```python
from build123d import *

# Parameters (mm, degrees)
CROQUIS1_W              = 900
CROQUIS1_H              = 1047
SALIENTE_EXTRUIR1_DEPTH = 2113
VACIADO2_T              = -10
CROQUIS2_W              = 880
CROQUIS2_H              = 2093
SALIENTE_EXTRUIR2_DEPTH = 5
CORTAR_EXTRUIR1_DEPTH   = 2
SALIENTE_EXTRUIR3_DEPTH = 300


with BuildPart() as part:
    # Croquis1 → Saliente-Extruir1 (new body)
    with BuildSketch(Plane(origin=(0, 0, 0), x_dir=(1, 0, 0), z_dir=(0, 1, 0))):
        Rectangle(CROQUIS1_W, CROQUIS1_H)
    extrude(amount=SALIENTE_EXTRUIR1_DEPTH)

    # Vaciado2
    vaciado2_openings = [part.faces().sort_by_distance(p)[0] for p in [
        (0, 1056.5, 523.5),
    ]]
    offset(amount=VACIADO2_T, openings=vaciado2_openings, kind=Kind.INTERSECTION)

    # Croquis2 → Saliente-Extruir2 (add)
    with BuildSketch(Plane.XY.offset(523.5)):
        with Locations((0, 1056.5)):
            Rectangle(CROQUIS2_W, CROQUIS2_H)
    extrude(amount=-SALIENTE_EXTRUIR2_DEPTH)

    # Croquis3 → Cortar-Extruir1 (cut)
    with BuildSketch(Plane.XY.offset(523.5)):
        Polygon((-136.509991439, 890.520139483), (155.469712472, 890.520139483), (9.479860517, 1243.170950701), align=None)
        Polygon((-63.176808732, 920.19459615), (-42.169545822, 1034.041849102), (9.479860517, 1064.169920858), (9.479860517, 1169.411963853), (65.966344659, 1064.169920858), (-12.532301764, 1019.623730372), (-63.176808732, 898.913148296), align=None, mode=Mode.SUBTRACT)
    extrude(amount=-CORTAR_EXTRUIR1_DEPTH, mode=Mode.SUBTRACT)

    # Croquis4 → Saliente-Extruir3 (add)
    with BuildSketch(Plane.XZ):
        with BuildLine():
            Line((-454.35645152, 548.5), (454.35645152, 548.5))
            ThreePointArc((454.35645152, 548.5), (468.953644638, 542.453644638), (475, 527.85645152))
            Line((475, 527.85645152), (475, -527.85645152))
            ThreePointArc((475, -527.85645152), (468.953644638, -542.453644638), (454.35645152, -548.5))
            Line((454.35645152, -548.5), (-454.35645152, -548.5))
            ThreePointArc((-454.35645152, -548.5), (-468.953644638, -542.453644638), (-475, -527.85645152))
            Line((-475, -527.85645152), (-475, 527.85645152))
            ThreePointArc((-475, 527.85645152), (-468.953644638, 542.453644638), (-454.35645152, 548.5))
        make_face()
    extrude(amount=SALIENTE_EXTRUIR3_DEPTH)


solid = part.part
```
Input: part model. Units: mm. Frame: model coordinates. A direction names the side the tool comes from. Give positions to 0.01 mm unless a question says otherwise; leave off trailing zeros. Write each loop counter-clockwise with the first axis right and the second up, starting at its lowest first coordinate (ties: lowest second). Pieces come first, ordered by that corner, then holes. Notation, with made-up numbers: (-16, 39) - (36, 39) arc R17 ccw to (36, 54) - close; hole circle Ø7 at (-17.5, -10). An arc over 180 degrees is marked (long way). Write item = value, one per line. Start each with the question number.
1) Material intervals for L1, parallel to Y at x = -322, z = -175.5; L2, parallel to Z at x = 327.5, y = 642; L3, parallel to X at y = 349, z = -102, sorted ascending. Write a range as [from, to].
2) Cut plane A-A (z = -320.5). Return loops of the section in (x, y), and give its area (3 significant figures).
3) Reachability of faces 1 (the face through (-6, 1042, -523.5)), 2 (the face through (-37.5, 960.11, 522.51)), 3 (the face through (-440, 1042, 10)) from +Z, -Z, +X, -X, +Y, -Y: full face, straight path, thin tool, end or side. Return the list, or none.
4) Draft query along X for faces 4 (the face through (-475, -148, -7)), 5 (the face through (1, 1045, 523.5)), 6 (the face through (-6, 10, -5)). Return one class per face: pulls with the +X half, pulls with the -X half, needs draft (parallel to the pull), parting line crosses it, or undercut.
5) Cut plane D-D (y = 1093). Return loops of the section in (x, z), and give its area (3 significant figures).
6) Cut plane C-C (y = 1627). Return loops of the section in (x, z).
7) Pin query (flat end, axial travel): pin 1 (5 mm diameter, centred on x = 247.5, y = 1348.5, fed in from +Z); pin 2 (4 mm diameter, centred on y = 872.5, z = -426.5, fed in from +X); pin 3 (8 mm diameter, centred on y = 323.5, z = 155.5, fed in from -X). Return the tip coordinate at first contact, or that it passes through.
8) Cut plane B-B (x = -410.5). Return loops of the section in (y, z).
Answers follow:
q1.L1 = [-300, 10], [2103, 2113]
q1.L2 = [-523.5, -513.5], [518.5, 523.5]
q1.L3 = [-450, -440], [440, 450]
q2.outline = (-475, -300) - (475, -300) - (475, 0) - (450, 0) - (450, 2113) - (-450, 2113) - (-450, 0) - (-475, 0) - close; hole (-440, 10) - (440, 10) - (440, 2103) - (-440, 2103) - close
q2.area = 345,000 mm^2
q3.face_1 = -Z, +X, -X, +Y
q3.face_2 = +Z
q3.face_3 = none
q4.face_4 = pulls with the -X half
q4.face_5 = needs draft
q4.face_6 = undercut
q5.outline = (-450, -523.5) - (450, -523.5) - (450, 523.5) - (71.65, 523.5) - (71.65, 521.5) - (50.49, 521.5) - (50.49, 523.5) - (9.48, 523.5) - (9.48, 521.5) - (-52.69, 521.5) - (-52.69, 523.5) - (-450, 523.5) - close; hole (-440, -513.5) - (440, -513.5) - (440, 518.5) - (-440, 518.5) - close
q5.area = 34,000 mm^2
q6.outline = (-450, -523.5) - (450, -523.5) - (450, 523.5) - (-450, 523.5) - close; hole (-440, -513.5) - (440, -513.5) - (440, 518.5) - (-440, 518.5) - close
q7.pin_1 = 523.5
q7.pin_2 = 450
q7.pin_3 = -450
q8.outline = (-300, -548.5) - (0, -548.5) - (0, -523.5) - (2113, -523.5) - (2113, 523.5) - (0, 523.5) - (0, 548.5) - (-300, 548.5) - close; hole (10, -513.5) - (2103, -513.5) - (2103, 518.5) - (10, 518.5) - close
